Here's how the part is built. I have some questions about the finished solid (model axes, mm). Give positions to 0.01 mm unless a question says otherwise; leave off trailing zeros. Loops run counter-clockwise (first coordinate to the right, second up) from the corner with the lowest first, then second, coordinate; pieces in that order, holes last. Notation, with made-up numbers: (-0.75, 16.25) -> (56.25, 16.25) arc R16 ccw to (56.25, 22.25) -> close; hole circle Ø6 at (-33.75, 74.5). An arc over 180 degrees is marked (long way). Answer in a Markdown table with one row per item. Add a question column.
Item 1: If we section it at C-C (x = -1): Write out the boundary of the cut face in (y, z), then the cut area to 3 significant figures.
Item 2: We'd pull the mould along Y, two halves only. Please class faces 1 (the face through (-1.5, 0.07, 3.45)), 2 (the face through (-1.3, -1.4, 7)), 3 (the face through (-1.36, 2.39, 3.45)), 4 (the face through (1.36, -2.39, 3.45)): released by +Y, released by -Y, zero draft, split by the parting line, or undercut.
Item 3: If we section it at D-D (y = 2.5): Write out the boundary of the cut face in (x, z), then the cut area to 3 significant figures.
Item 4: If we section it at A-A (z = 6): Write out the boundary of the cut face in (x, y).
Item 5: If I drill on line 1 (X direction, y = -1, z = 1.5); line 2 (X direction, y = -0.25, z = 6.5); line 3 (Y direction, x = -0.15, z = 2), over which ranges is the centre line in solid material (lowest first)?
Item 6: For P1, Ø2, axis at x = 2, z = 2.5, coming from the +Y side; P2, Ø1.5, axis at x = 0.5, z = 1.5, coming from the +Y side, each with a flat end and sliding along its axis, tell me the tip position at first contact or that it passes through.
Item 7: If we section it at B-B (y = 0): Write out the boundary of the cut face in (x, z).
```python
from build123d import *

# Parameters (mm, degrees)
F0_R     = 1.5
F1_DEPTH = 7
F2_DEPTH = 5


with BuildPart() as f1:
    # F0 (on Top) → F1 (new body)
    with BuildSketch(Plane.XY):
        Polygon((2.75, -1.587713), (2.75, 1.587713), (0, 3.175426), (-2.75, 1.587713), (-2.75, -1.587713), (0, -3.175426), align=None)
        Circle(F0_R, mode=Mode.SUBTRACT)
    extrude(amount=F1_DEPTH)

    # F0 (on Top) → F2 (cut)
    with BuildSketch(Plane.XY):
        Circle(F0_R)
    extrude(amount=F2_DEPTH, mode=Mode.SUBTRACT)


solid = f1.part
```
Recorded:
| question | item | result |
|---|---|---|
| 1 | outline | (-2.6, 0) -> (-1.12, 0) -> (-1.12, 7) -> (-2.6, 7) -> close; (1.12, 0) -> (2.6, 0) -> (2.6, 7) -> (1.12, 7) -> close |
| 1 | area | 20.7 mm^2 |
| 2 | face 1 | undercut |
| 2 | face 2 | zero draft |
| 2 | face 3 | released by +Y |
| 2 | face 4 | released by -Y |
| 3 | outline | (-1.17, 0) -> (1.17, 0) -> (1.17, 7) -> (-1.17, 7) -> close |
| 3 | area | 16.4 mm^2 |
| 4 | outline | (-2.75, -1.59) -> (0, -3.18) -> (2.75, -1.59) -> (2.75, 1.59) -> (0, 3.18) -> (-2.75, 1.59) -> close; hole circle Ø3 at (0, 0) |
| 5 | line 1 | x = -2.75 to -1.12, 1.12 to 2.75 |
| 5 | line 2 | x = -2.75 to -1.48, 1.48 to 2.75 |
| 5 | line 3 | y = -3.09 to -1.49, 1.49 to 3.09 |
| 6 | P1 | stops at y = 2.6 |
| 6 | P2 | stops at y = 3.18 |
| 7 | outline | (-2.75, 0) -> (-1.5, 0) -> (-1.5, 7) -> (-2.75, 7) -> close; (1.5, 0) -> (2.75, 0) -> (2.75, 7) -> (1.5, 7) -> close |
